Answer from the drawing. Dimensions are ordinates in mm from the lowest x, y and z of the part. Round coordinates to 2 decimals unless told otherwise and drop trailing zeros. Loops run counter-clockwise (first coordinate to the right, second up) from the corner with the lowest first, then second, coordinate; pieces in that order, holes last. Notation, with made-up numbers: M 89,-14 L 123,-14 A8 cw 123,-8 Z; hole C 11,82 d5. An arc over 180 degrees is marked long. One line per item, written item: value.
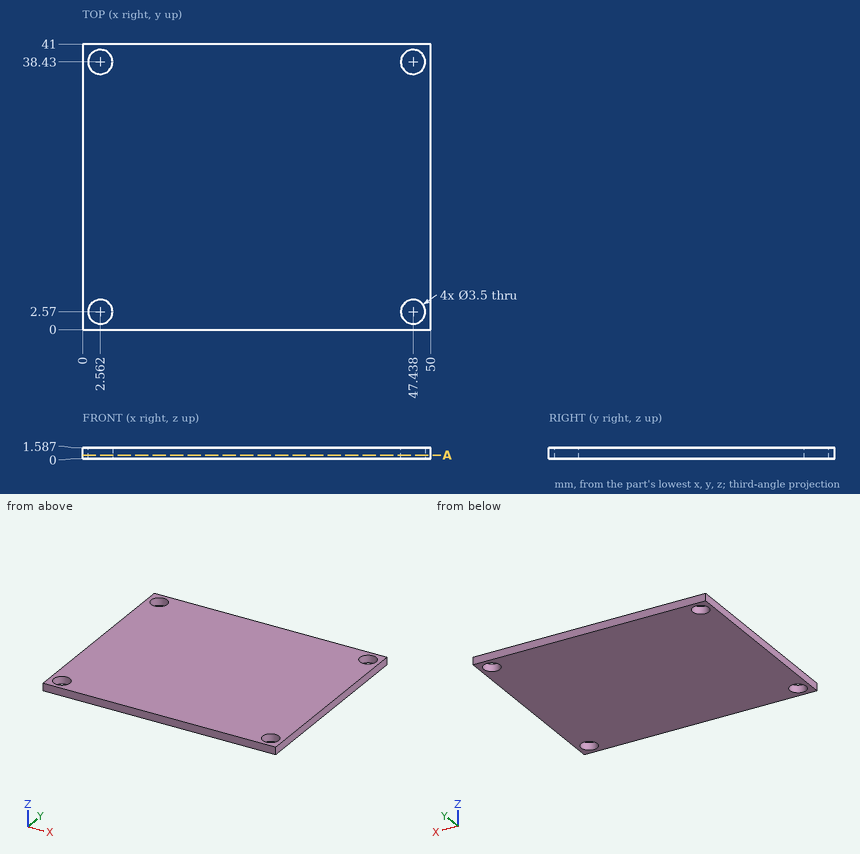
1) Find the intervals of material crossed by probe 1 along Y at (x, z) = (3.5, 0.1) (1 decimal); probe 2 along X at (y, z) = (3, 0.45) (1 decimal); probe 3 along Y at (x, z) = (4, 0.8) (1 decimal), in increasing order. Write a range as from..to.
Check values:
probe 1: 0..1.1, 4..37, 39.9..41
probe 2: 0..0.9, 4.3..45.7, 49.1..50
probe 3: 0..1.6, 3.6..37.4, 39.4..41
2) Find section A-A (z = 0.5). Give the vertices of the cut face in (x, y), then the cut area to 3 significant figures.
Check values:
outline: M 0,0 L 50,0 L 50,41 L 0,41 Z; hole C 2.56,2.57 d3.5; hole C 2.56,38.43 d3.5; hole C 47.44,2.57 d3.5; hole C 47.44,38.43 d3.5
area: 2,010 mm2
3) This flat-tipped pin is pushed along its axis until it touches: pin 1 (3 mm diameter, centred on x = 2.56, y = 38.43, fed in from +Z). Where does it stop, or does it pass through?
Check values:
pin 1: through
